from build123d import *

# Parameters (mm, degrees)
BOSS_EXTRUDE1_DEPTH = 3.175
SKETCH2_R           = 2.286
CUT_EXTRUDE1_DEPTH  = 133.001364813
FILLET1_R           = 1.5875


with BuildPart() as part:
    # Sketch1 → Boss-Extrude1 (new, symmetric)
    with BuildSketch(Plane(origin=(0, 0, 0), x_dir=(1, 0, 0), z_dir=(0, 1, 0))):
        with BuildLine():
            Line((0, 4.7625), (127, 4.7625))
            ThreePointArc((127, 4.7625), (131.7625, 0), (127, -4.7625))
            Line((127, -4.7625), (0, -4.7625))
            ThreePointArc((0, -4.7625), (-4.7625, 0), (0, 4.7625))
        make_face()
    extrude(amount=BOSS_EXTRUDE1_DEPTH, both=True)

    # Sketch2 → Cut-Extrude1 (cut, through all)
    with BuildSketch(Plane(origin=(0, 3.175, 0), x_dir=(1, 0, 0), z_dir=(0, 1, 0))):
        with Locations(Location((0, 0, 0), (0, 0, 270))):
            Circle(SKETCH2_R)
        with Locations(Location((127, 0, 0), (0, 0, 270))):
            Circle(SKETCH2_R)
    extrude(amount=-CUT_EXTRUDE1_DEPTH, mode=Mode.SUBTRACT)

    # Fillet1
    fillet1_edges = [part.edges().sort_by_distance(p)[0] for p in [
        (131.7625, 3.175, 0),
        (63.5, 3.175, -4.7625),
        (-4.7625, 3.175, 0),
        (63.5, -3.175, -4.7625),
        (131.7625, -3.175, 0),
        (63.5, -3.175, 4.7625),
        (-4.7625, -3.175, 0),
        (63.5, 3.175, 4.7625),
    ]]
    fillet(fillet1_edges, radius=FILLET1_R)


solid = part.part
Here's how the part is built. I have some questions about the finished solid (model axes, mm). Round coordinates to 2 decimals unless told otherwise and drop trailing zeros. Loops run counter-clockwise (first coordinate to the right, second up) from the corner with the lowest first, then second, coordinate; pieces in that order, holes last.
1. For P1, Ø3, axis at x = 43, y = 2, coming from the -Z side, with a flat end and sliding along its axis, tell me the tip position at first contact or that it passes through.
Answer list:
P1: stops at z = -4.76
2. We'd pull the mould along Z, two halves only. Please class faces 1 (the face through (64, 3.175, 0)), 2 (the face through (63, 0, -4.762)), 3 (the face through (-2.03, 0.04, 1.05)), 4 (the face through (-4.76, 0.02, 0.1)): +Z half, -Z half, draft (parallel to the pull), parting line (faces both ways), or undercut.
Answer list:
face 1: draft
face 2: -Z half
face 3: undercut
face 4: parting line
3. If I drill on line 1 along X through (y, z) = (0.75, 0); line 2 along X through (y, z) = (1, 1); line 3 along Z through (x, y) = (100, -1.75), over which ranges is the centre line in solid material (lowest first)?
Answer list:
line 1: x = -4.76 to -2.29, 2.29 to 124.71, 129.29 to 131.76
line 2: x = -4.66 to -2.06, 2.06 to 124.94, 129.06 to 131.66
line 3: z = -4.75 to 4.75
4. If we section it at C-C on z = 0: Write out the boundary of the cut face in (x, y) (1 decimal).
Answer list:
outline: (-4.8, -1.6) arc R1.6 ccw to (-3.2, -3.2) - (-2.3, -3.2) - (-2.3, 3.2) - (-3.2, 3.2) arc R1.6 ccw to (-4.8, 1.6) - close; (2.3, -3.2) - (124.7, -3.2) - (124.7, 3.2) - (2.3, 3.2) - close; (129.3, -3.2) - (130.2, -3.2) arc R1.6 ccw to (131.8, -1.6) - (131.8, 1.6) arc R1.6 ccw to (130.2, 3.2) - (129.3, 3.2) - close
5. If we section it at A-A on x = 74: Write out the boundary of the cut face in (y, z) (1 decimal), plus the area to 3 significant figures.
Answer list:
outline: (-3.2, -3.2) arc R1.6 ccw to (-1.6, -4.8) - (1.6, -4.8) arc R1.6 ccw to (3.2, -3.2) - (3.2, 3.2) arc R1.6 ccw to (1.6, 4.8) - (-1.6, 4.8) arc R1.6 ccw to (-3.2, 3.2) - close
area: 58.3 mm2
6. If we section it at B-B on y = -0.25: Write out the boundary of the cut face in (x, z) (1 decimal).
Answer list:
outline: (0, -4.8) - (127, -4.8) arc R4.8 ccw to (127, 4.8) - (0, 4.8) arc R4.8 ccw to start; hole circle Ø4.6 at (0, 0); hole circle Ø4.6 at (127, 0)
